from build123d import *

# Parameters (mm, degrees)
SKETCH2_R           = 8
SKETCH2_R_2         = 5
EXTRUDE_THIN1_DEPTH = 10
CUT_EXTRUDE1_DEPTH  = 10
SKETCH4_W           = 10
SKETCH4_H           = 10
BOSS_EXTRUDE1_DEPTH = 2
SKETCH5_R           = 3
CUT_EXTRUDE2_DEPTH  = 2
SKETCH6_W           = 25
SKETCH6_H           = 2.057623051
BOSS_EXTRUDE2_DEPTH = 2
SKETCH7_R           = 0.8
CUT_EXTRUDE3_DEPTH  = 2


with BuildPart() as part:
    # Sketch2 → Extrude-Thin1 (new body)
    with BuildSketch(Plane(origin=(0, 0, 0), x_dir=(1, 0, 0), z_dir=(0, 1, 0))):
        Circle(SKETCH2_R)
        Circle(SKETCH2_R_2, mode=Mode.SUBTRACT)
    extrude(amount=EXTRUDE_THIN1_DEPTH)

    # Sketch3 → Cut-Extrude1 (cut)
    with BuildSketch(Plane(origin=(0, 10, 0), x_dir=(1, 0, 0), z_dir=(0, 1, 0))):
        with BuildLine():
            Line((-8, 0), (8, 0))
            ThreePointArc((8, 0), (0, -8), (-8, 0))
        make_face()
    extrude(amount=-CUT_EXTRUDE1_DEPTH, mode=Mode.SUBTRACT)

    # Sketch4 → Boss-Extrude1 (add)
    with BuildSketch(Plane.XY):
        with Locations((10, 5)):
            Rectangle(SKETCH4_W, SKETCH4_H)
        with Locations((-10, 5)):
            Rectangle(SKETCH4_W, SKETCH4_H)
    extrude(amount=BOSS_EXTRUDE1_DEPTH)

    # Sketch5 → Cut-Extrude2 (cut)
    with BuildSketch(Plane(origin=(0, 0, 0), x_dir=(-1, 0, 0), z_dir=(0, 0, -1))):
        with Locations((-11.674262076, 5.406814048)):
            Circle(SKETCH5_R)
        with Locations((11.885931395, 5.406814048)):
            Circle(SKETCH5_R)
    extrude(amount=-CUT_EXTRUDE2_DEPTH, mode=Mode.SUBTRACT)

    # Sketch6 → Boss-Extrude2 (add)
    with BuildSketch(Plane(origin=(0, 10, 0), x_dir=(1, 0, 0), z_dir=(0, 1, 0))):
        with Locations((-20.5, -1.028811526)):
            Rectangle(SKETCH6_W, SKETCH6_H)
    extrude(amount=BOSS_EXTRUDE2_DEPTH)

    # Sketch7 → Cut-Extrude3 (cut)
    with BuildSketch(Plane(origin=(0, 12, 0), x_dir=(1, 0, 0), z_dir=(0, 1, 0))):
        with Locations((-31.5, -1.029261487)):
            Circle(SKETCH7_R)
    extrude(amount=-CUT_EXTRUDE3_DEPTH, mode=Mode.SUBTRACT)


solid = part.part
Read the model definition and answer for the solid it produces. Units are mm, in the model's axes. A direction names the side the tool comes from. Coordinates: 2 decimals unless noted, no trailing zeros. Loops run counter-clockwise (first coordinate to the right, second up) from the corner with the lowest first, then second, coordinate; pieces in that order, holes last. Notation, with made-up numbers: (1.25, 67.25) -> (9.25, 67.25) arc R28 cw to (9.25, 99.25) -> close; hole circle Ø3 at (-12.75, 30.5). An arc over 180 degrees is marked (long way). Write item = value, one per line. Start each with the question number.
1) The part is cut by section C-C, the plane y = 1.5. Determine the outline of the cut face in (x, z), plus the area to 3 significant figures.
2) The part is cut by section B-B, the plane y = 6.5. Determine the outline of the cut face in (x, z), plus the area to 3 significant figures.
3) The part is cut by section D-D, the plane z = -2. Determine the outline of the cut face in (x, y), plus the area to 3 significant figures.
4) The part is cut by section A-A, the plane x = -31.5. Determine the outline of the cut face in (y, z), plus the area to 3 significant figures.
5) For faces 1 (the face through (-9, 4, 2)), 2 (the face through (3.3, 10, -4.2)), 3 (the face through (-14, 8, 0)), 4 (the face through (-15, 4.9, 1)), 5 (the face through (-5, 5, 1)), determine the directions among +Z, -Z, +X, -X, +Y, -Y from which every point of the face is accessible in a straight line to the end or side of a thin tool.
6) Find the intervals of material crossed by L1, parallel to X at y = 8.25, z = -0.25; L2, parallel to X at y = 2, z = 1.25; L3, parallel to X at y = 6, z = 1.5, in increasing order. Write a range as from..to.
7) Given P1, Ø5, axis at x = 11.5, y = 4.5, coming from the +Z side; P2, Ø4, axis at x = -22.5, z = -3, coming from the +Y side; P3, Ø2.5, axis at x = -31.5, z = 1.03, coming from the +Y side; P4, Ø0.6, axis at y = 10.5, z = 1, coming from the +X side, each flat-ended and moving along its own axis, determine where each tip first touches the part or whether it passes through.
8) The mould has two halves that part along Z. Classify faces 6 (the face through (-30.737, 11.014, 0.789)), 7 (the face through (5, 5, 1)), 8 (the face through (8.8, 4, 2)): pulls with the +Z half, pulls with the -Z half, needs draft (parallel to the pull), parting line crosses it, or undercut.
Result:
q1.outline = (-15, 0) -> (-8, 0) arc R8 ccw to (8, 0) -> (15, 0) -> (15, 2) -> (5, 2) -> (5, 0) arc R5 cw to (-5, 0) -> (-5, 2) -> (-15, 2) -> close
q1.area = 101 mm²
q2.outline = (-15, 0) -> (-14.68, 0) -> (-14.68, 2) -> (-15, 2) -> close; (-9.09, 0) -> (-8, 0) arc R8 ccw to (8, 0) -> (8.88, 0) -> (8.88, 2) -> (5, 2) -> (5, 0) arc R5 cw to (-5, 0) -> (-5, 2) -> (-9.09, 2) -> close; (14.47, 0) -> (15, 0) -> (15, 2) -> (14.47, 2) -> close
q2.area = 78.9 mm²
q3.outline = (-7.75, 0) -> (-4.58, 0) -> (-4.58, 10) -> (-7.75, 10) -> close; (4.58, 0) -> (7.75, 0) -> (7.75, 10) -> (4.58, 10) -> close
q3.area = 63.3 mm²
q4.outline = (10, 0) -> (12, 0) -> (12, 0.23) -> (10, 0.23) -> close; (10, 1.83) -> (12, 1.83) -> (12, 2.06) -> (10, 2.06) -> close
q4.area = 0.915 mm²
q5.face_1 = +Z, +X, -X, -Y
q5.face_2 = +Z, -Z, +X, +Y
q5.face_3 = -Z, -X, +Y, -Y
q5.face_4 = +Z, -Z, -X, -Y
q5.face_5 = +Z, +Y, -Y
q6.L1 = -8..-4.99, 4.99..8
q6.L2 = -15..-5, 5..15
q6.L3 = -15..-14.83, -8.95..-5, 5..8.73, 14.62..15
q7.P1 = 2
q7.P2 = through
q7.P3 = 12
q7.P4 = -8
q8.face_6 = undercut
q8.face_7 = needs draft
q8.face_8 = pulls with the +Z half
